from build123d import *

# Parameters (mm, degrees)
F0_R       = 152.4
F1_DEPTH   = 304.8
F2_R       = 146.05
F3_DEPTH   = 292.1
F4_R       = 0.0127
F5_DEPTH   = 177.8
F6_R       = 0.0127
F7_DEPTH   = 152.4
F8_R       = 146.05
F7_FACE1_R = 0.0127
F10_R      = 0.0127
F11_DEPTH  = 25.4
F12_R      = 12.7
F13_DEPTH  = 165.1
F14_R      = 19.05
F14_R_2    = 12.7
F15_DEPTH  = 114.3


with BuildPart() as f1:
    # F0 (on Top) → F1 (new body)
    with BuildSketch(Plane.XY):
        Circle(F0_R)
    extrude(amount=F1_DEPTH)

    # F2 (on face) → F3 (cut)
    with BuildSketch(Plane.XY.offset(304.8)):
        Circle(F2_R)
    extrude(amount=-F3_DEPTH, mode=Mode.SUBTRACT)

    # F4 (on face) → F5 (join)
    with BuildSketch(Plane(origin=(0, 0, 0), x_dir=(1, 0, 0), z_dir=(0, 0, -1))):
        with Locations((76.2, 0)):
            Circle(F4_R)
    extrude(amount=F5_DEPTH)

    # F6 (on face) → F7 (cut)
    with BuildSketch(Plane(origin=(0, 0, 0), x_dir=(1, 0, 0), z_dir=(0, 0, -1))):
        with Locations((76.2, 0)):
            Circle(F6_R)
    extrude(amount=F7_DEPTH, mode=Mode.SUBTRACT)

    # F8 (on face) → F9 section 0
    with BuildSketch(Plane(origin=(0, 0, 0), x_dir=(1, 0, 0), z_dir=(0, 0, -1))):
        Circle(F8_R)
    # F7_face1 (on face) → F9 section 1
    with BuildSketch(Plane(origin=(76.2, 0, -152.4), x_dir=(1, 0, 0), z_dir=(0, 0, 1))):
        Circle(F7_FACE1_R)
    loft()

    # F10 (on face) → F11 (cut)
    with BuildSketch(Plane(origin=(0, 0, -177.8), x_dir=(1, 0, 0), z_dir=(0, 0, -1))):
        with Locations((76.2, 0)):
            Circle(F10_R)
    extrude(amount=-F11_DEPTH, mode=Mode.SUBTRACT)

    # F12 (on face) → F13 (cut)
    with BuildSketch(Plane.XY.offset(12.7)):
        with Locations((-76.2, 0)):
            Circle(F12_R)
    extrude(amount=-F13_DEPTH, mode=Mode.SUBTRACT)

    # F14 (on face) → F15 (join)
    with BuildSketch(Plane.XY.offset(12.7)):
        with Locations((-76.2, 0)):
            Circle(F14_R)
        with Locations((-76.2, 0)):
            Circle(F14_R_2, mode=Mode.SUBTRACT)
    extrude(amount=F15_DEPTH)


solid = f1.part
Geometry: final body of the model. Coordinates: model frame, mm. A direction names the side the tool comes from. Coordinates: 2 decimals unless noted, no trailing zeros. Order: outer loops, then holes, each group sorted by start corner. A loop starts at its lowest first (then second) coordinate and runs counter-clockwise, first axis right, second up. Notation, with made-up numbers: (-10.75, 54) - (15.25, 54) arc R10 cw to (15.25, 73) - close; hole circle Ø10 at (70, 67). An arc over 180 degrees is marked (long way). Use one line per item in the form item = value.
1) Mould query, pull axis X, two halves, no side actions, for faces 3 (the face through (78.3, -123.5, 0)), 4 (the face through (-64.468, -4.864, 33.91)), 5 (the face through (-120.94, -92.73, 150.27)). Classes: +X half, -X half, draft (parallel to the pull), parting line (faces both ways), or undercut.
Solutions:
face_3 = draft
face_4 = undercut
face_5 = parting line
2) Set-up query: faces 1 (the face through (78.3, -123.5, 304.8)), 2 (the face through (139.306, 43.869, 160.795)). Return all of +Z, -Z, +X, -X, +Y, -Y with unobstructed straight access to the full face (end or side cutting, diameter ignored); none if empty.
Solutions:
face_1 = +Z, +X, -X, +Y, -Y
face_2 = +Z
3) Pin query (flat end, axial travel): pin 1 (8 mm diameter, centred on x = -43.5, y = -62, fed in from +Z); pin 2 (6 mm diameter, centred on y = -41.5, z = 65.5, fed in from +X); pin 3 (1.5 mm diameter, centred on x = 11, z = 113, fed in from +Y); pin 4 (23 mm diameter, centred on x = -76.2, y = 0, fed in from -Z). Return the tip coordinate at first contact, or that it passes through.
Solutions:
pin_1 = 12.7
pin_2 = 147.46
pin_3 = 152.05
pin_4 = through
4) Section B-B (z = 162.5). Return loops of the section in (x, y).
Solutions:
outline = circle Ø304.8 at (0, 0); hole circle Ø292.1 at (0, 0)
5) Ray query, L1, parallel to Y at x = 0, z = 125; L2, parallel to Y at x = -76, z = 24; L3, parallel to X at y = 88.5, z = 233.5. Return the intervals inside material, ascending.
Solutions:
L1 = -152.4 to -146.05, 146.05 to 152.4
L2 = -132.1 to -124.72, -19.05 to -12.7, 12.7 to 19.05, 124.72 to 132.1
L3 = -124.07 to -116.18, 116.18 to 124.07
6) Section A-A (z = 73.5). Return loops of the section in (x, y), then the cut area to 3 significant figures.
Solutions:
outline = circle Ø304.8 at (0, 0); circle Ø38.1 at (-76.2, 0); hole circle Ø292.1 at (0, 0); hole circle Ø25.4 at (-76.2, 0)
area = 6,590 mm^2
